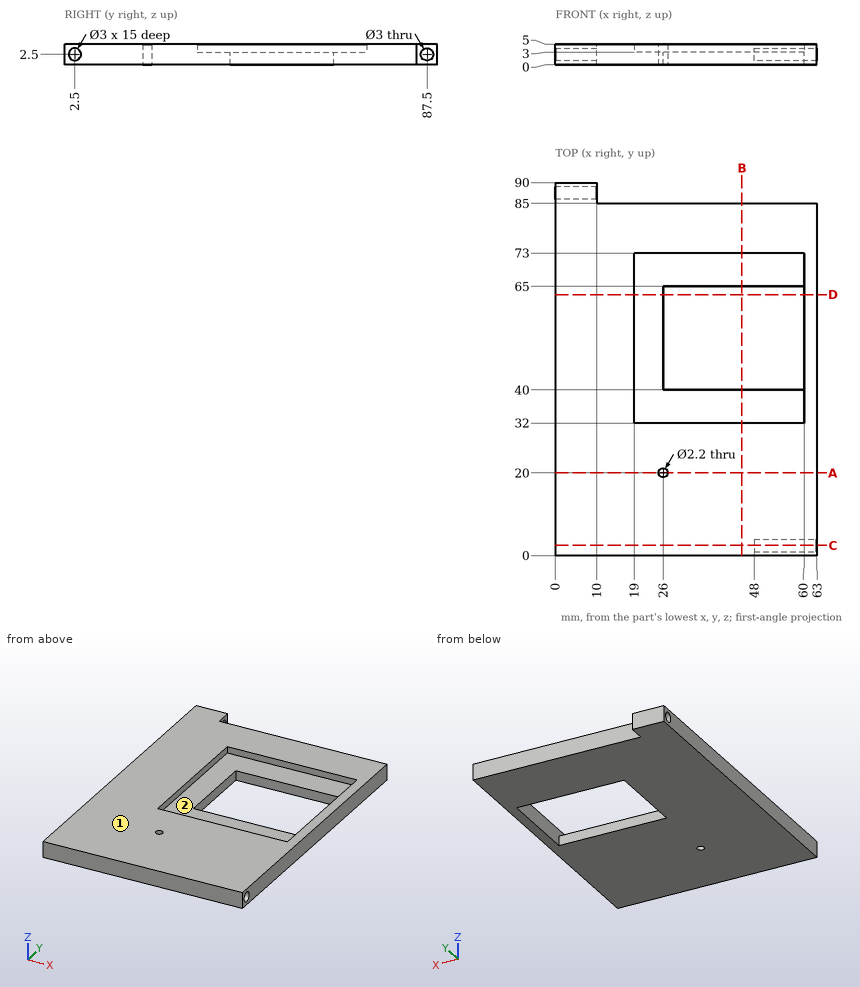
Can you work these out from the drawing? Everything is in mm from the part's minimum corner. Coordinates: 2 decimals unless noted, no trailing zeros. Order: outer loops, then holes, each group sorted by start corner. A loop starts at its lowest first (then second) coordinate and runs counter-clockwise, first axis right, second up. Notation, with made-up numbers: (30, 80.25) -> (57, 80.25) arc R28 ccw to (57, 112.25) -> close; hole circle Ø10 at (67, -20). An arc over 180 degrees is marked (long way). Use one line per item in the form item = value.
Q1. Imagine slicing it at D-D, the plane y = 63. List the corners of the cut face in (x, z) for me.
From the geometry:
outline = (0, 0) -> (26, 0) -> (26, 3) -> (19, 3) -> (19, 5) -> (0, 5) -> close; (60, 0) -> (63, 0) -> (63, 5) -> (60, 5) -> close
Q2. I need wall thicknesses on L1, parallel to Y at x = 24, z = 4.05; L2, parallel to Y at x = 26, z = 3.25; L3, parallel to Y at x = 2, z = 2.5. Which ranges of each line are inside material? Lowest first, please.
From the geometry:
L1 = 0 to 32, 73 to 85
L2 = 0 to 18.9, 21.1 to 32, 73 to 85
L3 = 0 to 86, 89 to 90
Q3. Imagine slicing it at C-C, the plane y = 2.5. List the corners of the cut face in (x, z) for me.
From the geometry:
outline = (0, 0) -> (63, 0) -> (63, 1) -> (48, 1) -> (48, 4) -> (63, 4) -> (63, 5) -> (0, 5) -> close
Q4. Imagine slicing it at B-B, the plane x = 45. List the corners of the cut face in (y, z) for me, then the cut area to 3 significant figures.
From the geometry:
outline = (0, 0) -> (40, 0) -> (40, 3) -> (32, 3) -> (32, 5) -> (0, 5) -> close; (65, 0) -> (85, 0) -> (85, 5) -> (73, 5) -> (73, 3) -> (65, 3) -> close
area = 268 mm²
Q5. We'd pull the mould along Y, two halves only. Please class the marked faces 1 and 2: released by +Y, released by -Y, zero draft, split by the parting line, or undercut.
From the geometry:
face_1 = zero draft
face_2 = undercut
Q6. Will these pins go through, and if not, where does the flat tip stop? P1, Ø1.5, axis at x = 35, z = 2, coming from the +Y side; P2, Ø2, axis at y = 37, z = 1, coming from the -X side; P3, Ø2.5, axis at y = 2.5, z = 2.5, coming from the +X side; P4, Ø2.5, axis at y = 87.5, z = 3.5, coming from the +X side.
From the geometry:
P1 = 85
P2 = 0
P3 = 48
P4 = 10
Q7. Imagine slicing it at A-A, the plane y = 20. List the corners of the cut face in (x, z) for me.
From the geometry:
outline = (0, 0) -> (24.9, 0) -> (24.9, 5) -> (0, 5) -> close; (27.1, 0) -> (63, 0) -> (63, 5) -> (27.1, 5) -> close
